```python
from build123d import *

# Parameters (mm, degrees)
F0_W     = 25.4
F0_H     = 25.4
F1_DEPTH = 25.4
F2_R     = 2.54
F3_W     = 2.54
F3_H     = 12.7
F3_R     = 1.27
F4_DEPTH = 1.27


with BuildPart() as f1:
    # F0 (on Top) → F1 (new body)
    with BuildSketch(Plane.XY):
        with Locations((2.765542, -3.050883)):
            Rectangle(F0_W, F0_H)
    extrude(amount=F1_DEPTH)

    # F2
    f2_edges = [f1.edges().sort_by_distance(p)[0] for p in [
        (2.765542, -15.750883, 25.4),
        (15.465542, -3.050883, 25.4),
        (15.465542, -15.750883, 12.7),
        (15.465542, -3.050883, 0),
        (2.765542, -15.750883, 0),
        (-9.934458, -15.750883, 12.7),
        (-9.934458, -3.050883, 0),
        (2.765542, 9.649117, 0),
        (2.765542, 9.649117, 25.4),
        (-9.934458, -3.050883, 25.4),
        (-9.934458, 9.649117, 12.7),
        (15.465542, 9.649117, 12.7),
    ]]
    fillet(f2_edges, radius=F2_R)

    # F3 (on face) → F4 (cut)
    with BuildSketch(Plane.XY.offset(25.4)):
        with Locations((2.765542, -1.780883)):
            Rectangle(F3_W, F3_H)
        with Locations((2.765542, -10.670883)):
            Circle(F3_R)
    extrude(amount=-F4_DEPTH, mode=Mode.SUBTRACT)


solid = f1.part
```
Work out the finished part from the listing and answer in its coordinate system (mm). A direction names the side the tool comes from. Give positions to 0.01 mm unless a question says otherwise; leave off trailing zeros. Loops run counter-clockwise (first coordinate to the right, second up) from the corner with the lowest first, then second, coordinate; pieces in that order, holes last. Notation, with made-up numbers: (56, 32) -> (112, 32) arc R13 ccw to (112, 46) -> close; hole circle Ø4 at (7.25, 55.25). An arc over 180 degrees is marked (long way). Put each result on its own line as item: value. Start each with the question number.
Item 1: The part is cut by section C-C (x = 2). Give the vertices of the cut face in (y, z).
Item 2: Which of the six approach directions +Z, -Z, +X, -X, +Y, -Y give full straight-line access (tool end or side, diameter ignored) to faces 1 (the face through (14.74, -2.91, 24.64)), 2 (the face through (3, 4.569, 25))?
Item 3: The part is cut by section B-B (y = 8.25). Give the vertices of the cut face in (x, z), then the cut area to 3 significant figures.
Item 4: The mould has two halves that part along Y. Classify faces 3 (the face through (2.908, -15.027, 24.636)), 4 (the face through (1.83, -9.81, 24.77)), 5 (the face through (2.91, 8.92, 0.76)): released by +Y, released by -Y, zero draft, split by the parting line, or undercut.
Item 5: Each of these flat-tipped pins is pushed along its axis until it touches: P1, Ø0.6, axis at y = -4.5, z = 24.5, coming from the -X side; P2, Ø1.4, axis at y = -3.5, z = 24.5, coming from the +X side; P3, Ø1.3, axis at x = 2.5, y = -2.5, coming from the +Z side. Where does it stop, or does it pass through?
Item 6: The part is cut by section A-A (x = -8.5). Give the vertices of the cut face in (y, z), then the cut area to 3 significant figures.
Item 7: Find the intervals of material crossed by L1, parallel to Z at x = 2, y = -2.5; L2, parallel to X at y = -7.5, z = 2; L3, parallel to Z at x = 10.5, y = -14, in increasing order. Write a range as [from, to].
Answers below:
1. outline: (-15.75, 2.54) arc R2.54 ccw to (-13.21, 0) -> (7.11, 0) arc R2.54 ccw to (9.65, 2.54) -> (9.65, 22.86) arc R2.54 ccw to (7.11, 25.4) -> (4.57, 25.4) -> (4.57, 24.13) -> (-8.13, 24.13) -> (-8.13, 25.4) -> (-9.66, 25.4) -> (-9.66, 24.13) -> (-11.68, 24.13) -> (-11.68, 25.4) -> (-13.21, 25.4) arc R2.54 ccw to (-15.75, 22.86) -> close
2. face 1: +Z, +X, +Y, -Y
2. face 2: +Z
3. outline: (-9.66, 2.54) arc R2.27 ccw to (-7.39, 0.27) -> (12.93, 0.27) arc R2.27 ccw to (15.19, 2.54) -> (15.19, 22.86) arc R2.27 ccw to (12.93, 25.13) -> (-7.39, 25.13) arc R2.27 ccw to (-9.66, 22.86) -> close
3. area: 614 mm2
4. face 3: released by -Y
4. face 4: undercut
4. face 5: released by +Y
5. P1: x = -9.55
5. P2: x = 15.29
5. P3: z = 24.13
6. outline: (-15.5, 2.54) arc R2.29 ccw to (-13.21, 0.25) -> (7.11, 0.25) arc R2.29 ccw to (9.4, 2.54) -> (9.4, 22.86) arc R2.29 ccw to (7.11, 25.15) -> (-13.21, 25.15) arc R2.29 ccw to (-15.5, 22.86) -> close
6. area: 615 mm2
7. L1: [0, 24.13]
7. L2: [-9.88, 15.41]
7. L3: [0.13, 25.27]
